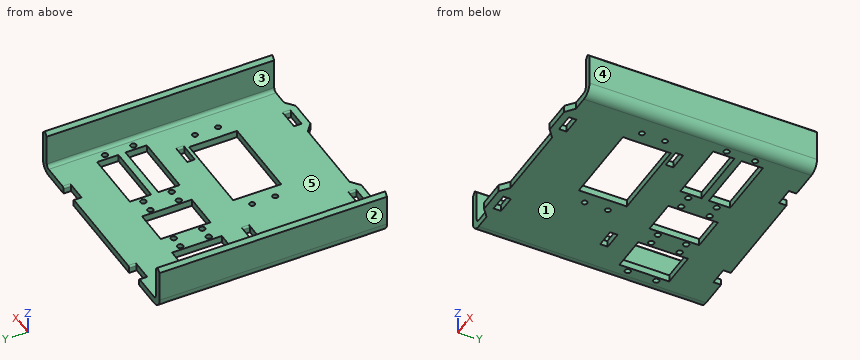
```python
from build123d import *

# Parameters (mm, degrees)
SKETCH_W          = 124.4
SKETCH_H          = 132
PAD_DEPTH         = 4
SKETCH001_W       = 4
SKETCH001_H       = 132
PAD001_DEPTH      = 19.6
PAD002_DEPTH      = 132
SKETCH003_W       = 10.5
SKETCH003_H       = 4.25
POCKET_DEPTH      = 4.001
POCKET_DEPTH_BACK = 21.601
FILLET_R          = 6
FILLET001_R       = 2
FILLET002_R       = 1
SKETCH004_R       = 1.6
SKETCH004_R_2     = 1.5
SKETCH004_W       = 20
SKETCH004_H       = 28
SKETCH004_W_2     = 35
SKETCH004_H_2     = 12
SKETCH004_W_3     = 47
SKETCH004_H_3     = 27
POCKET001_DEPTH   = 4.001


with BuildPart() as part:
    # Sketch → Pad (new body)
    with BuildSketch(Plane.XY):
        with Locations((0, 66)):
            Rectangle(SKETCH_W, SKETCH_H)
    extrude(amount=-PAD_DEPTH)

    # Sketch001 → Pad001 (join)
    with BuildSketch(Plane.XY):
        with Locations((-60.2, 66)):
            Rectangle(SKETCH001_W, SKETCH001_H)
        with Locations((60.2, 66)):
            Rectangle(SKETCH001_W, SKETCH001_H)
    extrude(amount=PAD001_DEPTH)

    # Sketch002 → Pad002 (join)
    with BuildSketch(Plane.XZ):
        Polygon((-58.2, 19.6), (-62.2, 19.6), (-60.2, 21.6), align=None)
        Polygon((58.2, 19.6), (62.2, 19.6), (60.2, 21.6), align=None)
    extrude(amount=-PAD002_DEPTH)

    # Sketch003 → Pocket (cut, two sides)
    with BuildSketch(Plane.XY) as pocket_sk:
        with Locations((-35, 6.125)):
            Rectangle(SKETCH003_W, SKETCH003_H)
        with Locations((-35, 66.125)):
            Rectangle(SKETCH003_W, SKETCH003_H)
        with Locations((-35, 129.875)):
            Rectangle(SKETCH003_W, SKETCH003_H)
        with Locations((35, 6.125)):
            Rectangle(SKETCH003_W, SKETCH003_H)
        with Locations((35, 66.125)):
            Rectangle(SKETCH003_W, SKETCH003_H)
        with Locations((35, 129.875)):
            Rectangle(SKETCH003_W, SKETCH003_H)
        Polygon((-42.75, 0), (-27.25, 0), (-22.25, 4), (22.25, 4), (27.25, 0), (42.75, 0), (47.75, 4), (90, 4), (90, -46), (-90, -46), (-90, 4), (-47.75, 4), align=None)
    extrude(amount=-POCKET_DEPTH, mode=Mode.SUBTRACT)
    extrude(pocket_sk.sketch, amount=POCKET_DEPTH_BACK, mode=Mode.SUBTRACT)

    # Fillet
    fillet_edges = [part.edges().sort_by_distance(p)[0] for p in [
        (-62.2, 68, -4),
        (62.2, 68, -4),
    ]]
    fillet(fillet_edges, radius=FILLET_R)

    # Fillet001
    fillet001_edges = [part.edges().sort_by_distance(p)[0] for p in [
        (-58.2, 68, 0),
        (58.2, 68, 0),
    ]]
    fillet(fillet001_edges, radius=FILLET001_R)

    # Fillet002
    fillet002_edges = [part.edges().sort_by_distance(p)[0] for p in [
        (-40.25, 129.875, 0),
        (-29.75, 129.875, 0),
        (29.75, 129.875, 0),
        (40.25, 129.875, 0),
        (29.75, 66.125, 0),
        (40.25, 66.125, 0),
        (29.75, 6.125, 0),
        (40.25, 6.125, 0),
        (-40.25, 6.125, 0),
        (-29.75, 6.125, 0),
        (-40.25, 66.125, 0),
        (-29.75, 66.125, 0),
    ]]
    fillet(fillet002_edges, radius=FILLET002_R)

    # Sketch004 → Pocket001 (cut, through all)
    with BuildSketch(Plane.XY):
        with Locations((-52.5, 102)):
            Circle(SKETCH004_R)
        with Locations((-27.5, 102)):
            Circle(SKETCH004_R)
        with Locations((-27.5, 86)):
            Circle(SKETCH004_R)
        with Locations((-52.5, 86)):
            Circle(SKETCH004_R)
        with Locations((-20.5, 102)):
            Circle(SKETCH004_R)
        with Locations((4.5, 102)):
            Circle(SKETCH004_R)
        with Locations((4.5, 86)):
            Circle(SKETCH004_R)
        with Locations((-20.5, 86)):
            Circle(SKETCH004_R)
        with Locations((12, 102)):
            Circle(SKETCH004_R)
        with Locations((53, 102)):
            Circle(SKETCH004_R)
        with Locations((12, 86)):
            Circle(SKETCH004_R)
        with Locations((53, 86)):
            Circle(SKETCH004_R)
        with Locations((46, 55)):
            Circle(SKETCH004_R_2)
        with Locations((46, 42)):
            Circle(SKETCH004_R_2)
        with Locations((-15, 55)):
            Circle(SKETCH004_R_2)
        with Locations((-15, 42)):
            Circle(SKETCH004_R_2)
        with Locations((-40, 94)):
            Rectangle(SKETCH004_W, SKETCH004_H)
        with Locations((-8, 94)):
            Rectangle(SKETCH004_W, SKETCH004_H)
        with Locations((32.5, 102)):
            Rectangle(SKETCH004_W_2, SKETCH004_H_2)
        with Locations((32.5, 86)):
            Rectangle(SKETCH004_W_2, SKETCH004_H_2)
        with Locations((15.5, 48.5)):
            Rectangle(SKETCH004_W_3, SKETCH004_H_3)
    extrude(amount=-POCKET001_DEPTH, mode=Mode.SUBTRACT)


solid = part.part
```
CAD build for the part. Positions are in the model's coordinates, mm. Face numbers are marked on the shaded views. A direction names the side the tool comes from. Coordinates: 2 decimals unless noted, no trailing zeros. Order: outer loops, then holes, each group sorted by start corner. A loop starts at its lowest first (then second) coordinate and runs counter-clockwise, first axis right, second up.
(1) Saw through at C-C, the plane x = -52.5. Write the cut outline in (y, z), and give its area (3 significant figures).
Solution:
outline: (4, -4) - (84.4, -4) - (84.4, 0) - (4, 0) - close; (87.6, -4) - (100.4, -4) - (100.4, 0) - (87.6, 0) - close; (103.6, -4) - (132, -4) - (132, 0) - (103.6, 0) - close
area: 486 mm2
(2) Pin check, flat tips, straight feed: pin 1 Ø3.5 at (y, z) = (66.5, -2.5) entering from +X; pin 2 Ø3 at (x, y) = (-27.5, 86) entering from +Z; pin 3 Ø12 at (x, z) = (-12, 1) entering from -Y; pin 4 Ø2 at (y, z) = (45.5, -2) entering from +X. Stop position of each tip, or through.
Solution:
pin 1: stops at x = 61.53
pin 2: passes through
pin 3: stops at y = 4
pin 4: stops at x = 61.4
(3) Mould opens along X. For the marked faces 1, 2 and 3 say: released by +X, released by -X, zero draft, split by the parting line, or undercut.
Solution:
face 1: zero draft
face 2: released by -X
face 3: undercut
(4) Drill centre lines: L1, parallel to Y at x = -20.5, z = -3.05; L2, parallel to Y at x = -15, z = -1.1; L3, parallel to Y at x = 4.5, z = -0.95. Where is each one in solid material? Low to high.
Solution:
L1: y = 4 to 84.4, 87.6 to 100.4, 103.6 to 132
L2: y = 4 to 40.5, 43.5 to 53.5, 56.5 to 80, 108 to 132
L3: y = 4 to 35, 62 to 84.4, 87.6 to 100.4, 103.6 to 132
(5) Saw through at D-D, the plane z = 8.25. Write the cut outline in (x, y), and give its area (3 significant figures).
Solution:
outline: (-62.2, 4) - (-58.2, 4) - (-58.2, 132) - (-62.2, 132) - close; (58.2, 4) - (62.2, 4) - (62.2, 132) - (58.2, 132) - close
area: 1,020 mm2
(6) Saw through at B-B, the plane y = 42. Write the cut outline in (x, z).
Solution:
outline: (-62.2, 2) arc R6 ccw to (-56.2, -4) - (-16.5, -4) - (-16.5, 0) - (-56.2, 0) arc R2 cw to (-58.2, 2) - (-58.2, 19.6) - (-60.2, 21.6) - (-62.2, 19.6) - close; (-13.5, -4) - (-8, -4) - (-8, 0) - (-13.5, 0) - close; (39, -4) - (44.5, -4) - (44.5, 0) - (39, 0) - close; (47.5, -4) - (56.2, -4) arc R6 ccw to (62.2, 2) - (62.2, 19.6) - (60.2, 21.6) - (58.2, 19.6) - (58.2, 2) arc R2 cw to (56.2, 0) - (47.5, 0) - close
(7) Saw through at A-A, the plane x = 12. Write the cut outline in (y, z), and give its area (3 significant figures).
Solution:
outline: (4, -4) - (35, -4) - (35, 0) - (4, 0) - close; (62, -4) - (84.4, -4) - (84.4, 0) - (62, 0) - close; (87.6, -4) - (100.4, -4) - (100.4, 0) - (87.6, 0) - close; (103.6, -4) - (132, -4) - (132, 0) - (103.6, 0) - close
area: 378 mm2
(8) Which spindle directions (+Z, -Z, +X, -X, +Y, -Y) get a long thin tool onto all of the face, cutting with end or side? Do the marked faces 4 and 5. Say none if no direction does.
Solution:
face 4: +Z, -Z, +X, +Y, -Y
face 5: +Z, +Y, -Y
